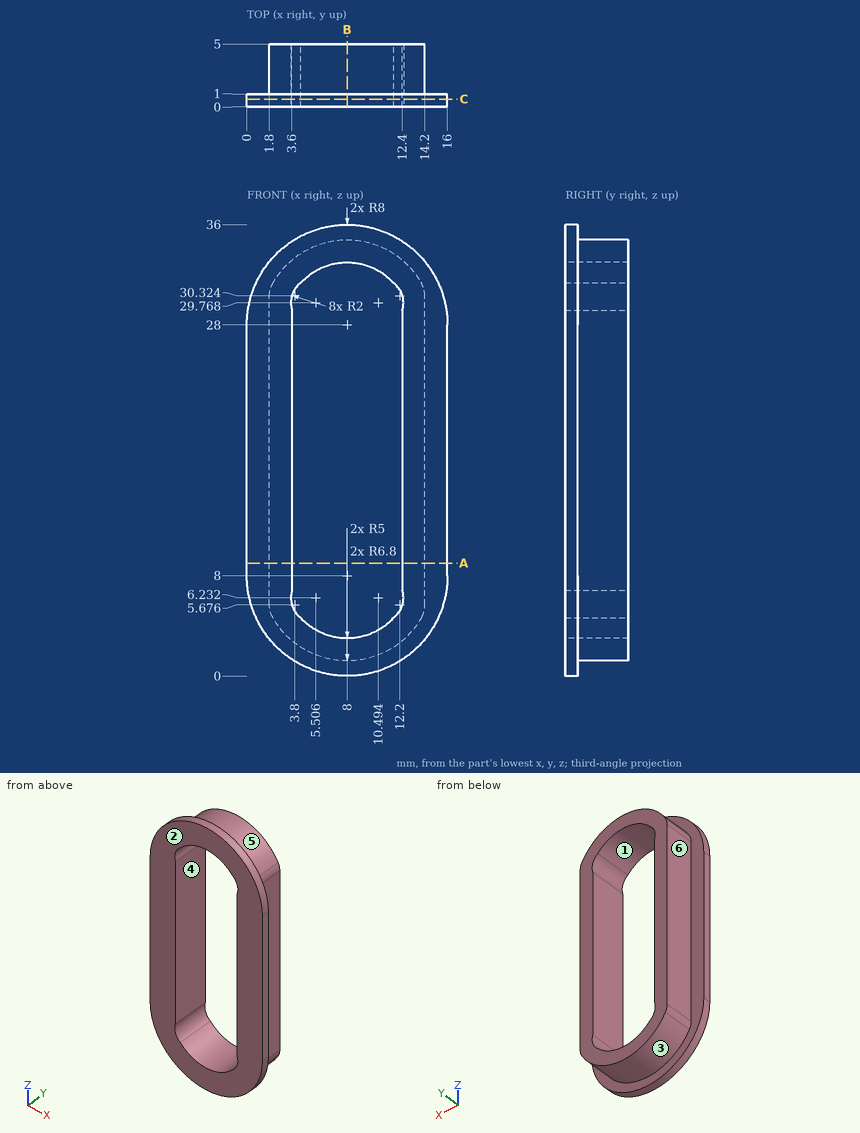
Verification items for this drawing (mm, ordinates from the low corner). A direction names the side the tool comes from. Coordinates: 2 decimals unless noted, no trailing zeros. Order: outer loops, then holes, each group sorted by start corner. A loop starts at its lowest first (then second) coordinate and runs counter-clockwise, first axis right, second up. Notation, with made-up numbers: M 85,69 L 137,69 A17 cw 137,77 Z; hole C 24.5,-13 d4. An arc over 180 degrees is marked long. Answer as a JSON object with one key per item and string values.
Q1. Cross-section at A-A on z = 9. Record the cut outline in (x, y), and give its area (3 significant figures).
Results are:
{"outline": "M 0,0 L 3.6,0 L 3.6,5 L 1.8,5 L 1.8,1 L 0,1 Z; M 12.4,0 L 16,0 L 16,1 L 14.2,1 L 14.2,5 L 12.4,5 Z", "area": "21.6 mm²"}
Q2. Tool access check on the marked faces 1, 2 and 3. Record the directions out of +Z, -Z, +X, -X, +Y, -Y that give a thin tool (end or side, any length) a straight path to the whole face; none if there is none.
Results are:
{"face 1": "+Y, -Y", "face 2": "+Z, -Z, +X, -X, -Y", "face 3": "-Z, +Y"}
Q3. Scan lines: line 1 (X direction, y = 2.6, z = 12); line 2 (X direction, y = 0.4, z = 4.5) (1 decimal); line 3 (Z direction, x = 7, y = 1.6) (1 decimal). Record each from-to range of solid material in increasing order.
Results are:
{"line 1": "x = 1.8 to 3.6, 12.4 to 14.2", "line 2": "x = 0.8 to 4.4, 11.6 to 15.2", "line 3": "z = 1.3 to 3.1, 32.9 to 34.7"}
Q4. Depth check by flat-ended pin: pin 1 Ø2.5 at (y, z) = (2.5, 15) entering from -X; pin 2 Ø2.5 at (y, z) = (2.5, 13.5) entering from +X; pin 3 Ø1 at (x, y) = (14, 4) entering from +Z. Enter the tip coordinate at first touch or a pass-through.
Results are:
{"pin 1": "stops at x = 1.8", "pin 2": "stops at x = 14.2", "pin 3": "stops at z = 32"}
Q5. Cross-section at C-C on y = 0.6. Record the cut outline in (x, z) (1 decimal).
Results are:
{"outline": "M 0,8 A8 ccw 16,8 L 16,28 A8 ccw 0,28 Z; hole M 3.6,6.8 A2 ccw 4.3,4.6 A5 ccw 11.7,4.6 A2 ccw 12.4,6.8 L 12.4,29.2 A2 ccw 11.7,31.4 A5 ccw 4.3,31.4 A2 ccw 3.6,29.2 Z"}
Q6. Cross-section at B-B on x = 8. Record the cut outline in (y, z), and give its area (3 significant figures).
Results are:
{"outline": "M 0,0 L 1,0 L 1,1.2 L 5,1.2 L 5,3 L 0,3 Z; M 0,33 L 5,33 L 5,34.8 L 1,34.8 L 1,36 L 0,36 Z", "area": "20.4 mm²"}
Q7. Release check for a two-part mould opening along X. For the marked faces 4, 5 and 6 record: released by +X, released by -X, zero draft, split by the parting line, or undercut.
Results are:
{"face 4": "undercut", "face 5": "split by the parting line", "face 6": "released by -X"}
